Design review of the part built by this model. Coordinates are the model's own, in mm. Face numbers are marked on the shaded views. A direction names the side the tool comes from. Give positions to 0.01 mm unless a question says otherwise; leave off trailing zeros. Loops run counter-clockwise (first coordinate to the right, second up) from the corner with the lowest first, then second, coordinate; pieces in that order, holes last. Notation, with made-up numbers: (-5, -40) -> (13, -40) arc R11 cw to (13, -21) -> close; hole circle Ø1 at (30, 15.5). An arc over 180 degrees is marked (long way). Answer as CSV lines item,"result".
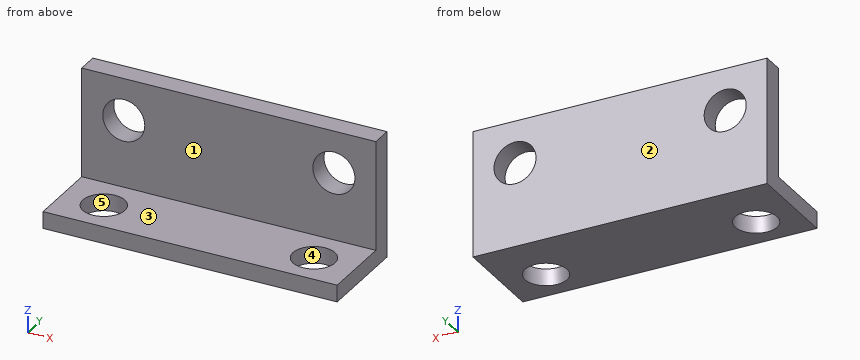
from build123d import *

# Parameters (mm, degrees)
F0_W     = 88.9
F0_H     = 33.02
F0_R     = 6.35
F1_DEPTH = 3.175
F0_H_2   = 5.08
F2_DEPTH = 25.4
F3_DEPTH = 3.175
F5_D     = 12.7


with BuildPart() as f1:
    # F0 (on Front) → F1 (new body, symmetric)
    with BuildSketch(Plane.XZ):
        with Locations((-26.614039, -3.81)):
            Rectangle(F0_W, F0_H)
        with Locations((-58.364039, 0)):
            Circle(F0_R, mode=Mode.SUBTRACT)
        with Locations((5.135961, 0)):
            Circle(F0_R, mode=Mode.SUBTRACT)
    extrude(amount=F1_DEPTH, both=True)

    # F0 (on Front) → F2 (join)
    with BuildSketch(Plane.XZ):
        with Locations((-26.614039, -22.86)):
            Rectangle(F0_W, F0_H_2)
    extrude(amount=F2_DEPTH)

    # F0 (on Front) → F3 (join)
    with BuildSketch(Plane.XZ):
        with Locations((-26.614039, -22.86)):
            Rectangle(F0_W, F0_H_2)
    extrude(amount=-F3_DEPTH)

    # F5 (through all)
    with Locations(Plane.XY):
        with Locations((-58.364039, -14.605), (5.135961, -14.605)):
            Hole(F5_D / 2)


solid = f1.part
Q1. The part is to be moulded in two halves that separate along X. For the marked faces 3, 4 and 5, say which applies: pulls with the +X half, pulls with the -X half, needs draft (parallel to the pull), parting line crosses it, or undercut.
Filled sheet:
face 3,"needs draft"
face 4,"undercut"
face 5,"undercut"
Q2. We need section A-A, the plane z = 0. State the section outline as (x, y) points (3 decimals).
Filled sheet:
outline,"(-71.064, -3.175) -> (-64.714, -3.175) -> (-64.714, 3.175) -> (-71.064, 3.175) -> close; (-52.014, -3.175) -> (-1.214, -3.175) -> (-1.214, 3.175) -> (-52.014, 3.175) -> close; (11.486, -3.175) -> (17.836, -3.175) -> (17.836, 3.175) -> (11.486, 3.175) -> close"
Q3. To check wall thickness, follow probe 1 along Z at (x, y) = (-59, -22.25); probe 2 along Y at (x, z) = (-18, 3) (3 decimals); probe 3 along X at (y, z) = (-19.75, -21). State the ranges of each line that lie inside material, in increasing order. Write a range as from..to.
Filled sheet:
probe 1,"z = -25.4..-20.32"
probe 2,"y = -3.175..3.175"
probe 3,"x = -71.06..-62.09, -54.64..1.41, 8.86..17.84"
Q4. We need section C-C, the plane x = -43. State the section outline as (y, z) points (3 decimals), and give its area (3 significant figures).
Filled sheet:
outline,"(-25.4, -25.4) -> (3.175, -25.4) -> (3.175, 12.7) -> (-3.175, 12.7) -> (-3.175, -20.32) -> (-25.4, -20.32) -> close"
area,"355 mm^2"
Q5. For the marked faces 1 and 2, list the 3-axis set-ups (+Z, -Z, +X, -X, +Y, -Y) from which the entire face can be reached by the end or side of a thin tool; tool diameter is ignored.
Filled sheet:
face 1,"+Z, +X, -X, -Y"
face 2,"+Z, -Z, +X, -X, +Y"
Q6. We need section B-B, the plane x = -63. State the section outline as (y, z) points (3 decimals), and give its area (3 significant figures).
Filled sheet:
outline,"(-25.4, -25.4) -> (-18.944, -25.4) -> (-18.944, -20.32) -> (-25.4, -20.32) -> close; (-10.266, -25.4) -> (3.175, -25.4) -> (3.175, -4.339) -> (-3.175, -4.339) -> (-3.175, -20.32) -> (-10.266, -20.32) -> close; (-3.175, 4.339) -> (3.175, 4.339) -> (3.175, 12.7) -> (-3.175, 12.7) -> close"
area,"256 mm^2"
Q7. Clearance check with flat-ended pins moving along their axes: pin 1 Ø2 at (x, z) = (-20.5, 5) entering from -Y (3 decimals); pin 2 Ø8 at (y, z) = (-9, 4) entering from +X. State where each tip first meets the part, or that it passes through.
Filled sheet:
pin 1,"stops at y = -3.175"
pin 2,"passes through"
Q8. We need section D-D, the plane z = 9.5. State the section outline as (x, y) points (3 decimals), and give its area (3 significant figures).
Filled sheet:
outline,"(-71.064, -3.175) -> (17.836, -3.175) -> (17.836, 3.175) -> (-71.064, 3.175) -> close"
area,"565 mm^2"
